from build123d import *

# Parameters (mm, degrees)
F0_R             = 45
F0_R_2           = 33
F1_DEPTH         = 17
F2_R             = 5
F3_DEPTH         = 0.5
F3_COPIES_COUNT  = 6
F6_DEPTH         = 10
F8_COUNT         = 6
F9_W             = 6
F9_H             = 9
F10_DEPTH        = 17
F10_COPIES_COUNT = 3
F12_DEPTH        = 10
F12_COPIES_COUNT = 3
F14_DEPTH        = 1
F14_COPIES_COUNT = 3


# Not quite as in the source:
# - a pattern or mirror of a feature is missing from the dataset's text; its kind, count and spacing are read off the source's solid
# - a feature names something its author has since deleted; it is built from what else it names


with BuildPart() as f1:
    # F0 (on Front) → F1 (new body)
    with BuildSketch(Plane.XZ):
        Circle(F0_R)
        Circle(F0_R_2, mode=Mode.SUBTRACT)
    extrude(amount=F1_DEPTH)

    # F2 (on Front) → F3 (cut)
    with BuildSketch(Plane.XZ):
        with Locations((0, 39)):
            Circle(F2_R)
    f3 = extrude(amount=F3_DEPTH, mode=Mode.SUBTRACT)

    # F3_copies: F3 ×6 about axis
    f3_copies_axis = Axis((0, 0, 0), (0, 1, 0))
    for i in range(1, F3_COPIES_COUNT):
        add(f3.rotate(f3_copies_axis, i * 360 / F3_COPIES_COUNT), mode=Mode.SUBTRACT)

    # F5 (on face) → F6 (cut)
    with BuildSketch(Plane.XZ.offset(17)):
        with BuildLine():
            Line((-30.5409561082, 12.5), (-43.2290411645, 12.5))
            ThreePointArc((-43.2290411645, 12.5), (-45, 0), (-43.2290411645, -12.5))
            Line((-43.2290411645, -12.5), (-30.5409561082, -12.5))
            ThreePointArc((-30.5409561082, -12.5), (-33, 0), (-30.5409561082, 12.5))
        make_face()
    f6 = extrude(amount=-F6_DEPTH, mode=Mode.SUBTRACT)

    # F8: F6 ×6 about axis
    f8_axis = Axis((0, -20.116, 0), (0, -1, 0))
    for i in range(1, F8_COUNT):
        add(f6.rotate(f8_axis, i * 360 / F8_COUNT), mode=Mode.SUBTRACT)

    # F9 (on face) → F10 (join)
    with BuildSketch(Plane.XZ.offset(7)):
        with Locations((42, 0)):
            Rectangle(F9_W, F9_H)
    f10 = extrude(amount=F10_DEPTH)

    # F10_copies: F10 ×3 about axis
    f10_copies_axis = Axis((0, 0, 0), (0, 1, 0))
    for i in range(1, F10_COPIES_COUNT):
        add(f10.rotate(f10_copies_axis, i * 360 / F10_COPIES_COUNT))

    # F11 (on face) → F12 (cut)
    with BuildSketch(Plane(origin=(0, 0, -4.5), x_dir=(1, 0, 0), z_dir=(0, 0, -1))):
        Polygon((39, 24), (39, 23.6), (43, 22), (43, 21), (41, 20), (41, 7), (44.7744346698, 7), (45, 7), (45, 24), align=None)
    f12 = extrude(amount=-F12_DEPTH, mode=Mode.SUBTRACT)

    # F12_copies: F12 ×3 about axis
    f12_copies_axis = Axis((0, 0, 0), (0, 1, 0))
    for i in range(1, F12_COPIES_COUNT):
        add(f12.rotate(f12_copies_axis, i * 360 / F12_COPIES_COUNT), mode=Mode.SUBTRACT)

    # F13 (on Top) → F14 (join, symmetric)
    with BuildSketch(Plane.XY):
        Polygon((37, -7), (39, -17), (39, -7), align=None)
    f14 = extrude(amount=F14_DEPTH, both=True)

    # F14_copies: F14 ×3 about axis
    f14_copies_axis = Axis((0, 0, 0), (0, 1, 0))
    for i in range(1, F14_COPIES_COUNT):
        add(f14.rotate(f14_copies_axis, i * 360 / F14_COPIES_COUNT))


solid = f1.part
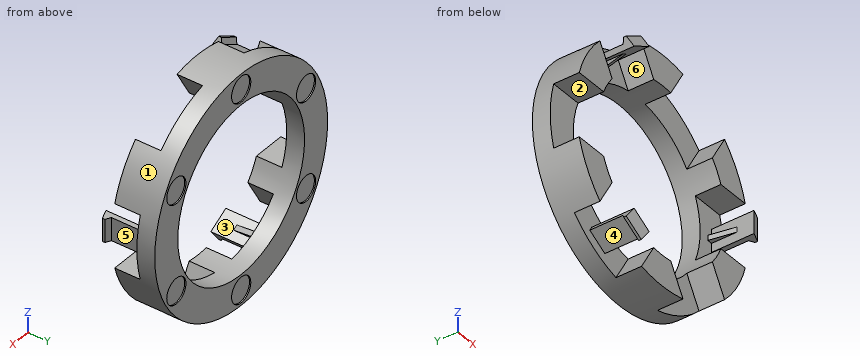
Source: CAD feature listing. Evaluate the final solid. Frame: model axes, mm. Face numbers are marked on the shaded views. A direction names the side the tool comes from. Give positions to 0.01 mm unless a question says otherwise; leave off trailing zeros. Order: outer loops, then holes, each group sorted by start corner. A loop starts at its lowest first (then second) coordinate and runs counter-clockwise, first axis right, second up. Notation, with made-up numbers: (57, -17.75) -> (105, -17.75) arc R23 ccw to (105, -6.75) -> close; hole circle Ø9 at (79.5, -8.75). An arc over 180 degrees is marked (long way). Write item = value, one per line.
Item 1: Ray query, probe 1 along Z at (x, y) = (0, -0.05); probe 2 along Y at (x, z) = (29, -30.5); probe 3 along Z at (x, y) = (17, -2.5). Return the intervals inside material, ascending.
Check result:
probe_1 = -45 to -44, -34 to -33, 33 to 34, 44 to 45
probe_2 = -7 to 0
probe_3 = -41.67 to -28.28, 28.28 to 41.67
Item 2: Section query B-B (z = -6.5). Output: boundary loops of the cut face in (x, y), then the cut area to 3 significant figures.
Check result:
outline = (-44.53, -7) -> (-32.35, -7) -> (-32.35, 0) -> (-44.53, 0) -> close; (32.35, -7) -> (44.53, -7) -> (44.53, 0) -> (32.35, 0) -> close
area = 170 mm²
Item 3: Set-up query: the marked faces 4, 5 and 6. Return all of +Z, -Z, +X, -X, +Y, -Y with unobstructed straight access to the full face (end or side cutting, diameter ignored); none if empty.
Check result:
face_4 = -Z, -X
face_5 = +X
face_6 = -Y
Item 4: Contact query for flat-ended pins moving along their axis: pin 1 (10 mm diameter, centred on x = -2, z = 40.5, fed in from -Y); pin 2 (3 mm diameter, centred on x = 41, y = -15.5, fed in from +Z); pin 3 (1 mm diameter, centred on x = -8.5, y = -16, fed in from +Z); pin 4 (11 mm diameter, centred on x = 1.5, z = -38.5, fed in from +Y). Output: stop coordinate, or through.
Check result:
pin_1 = -17
pin_2 = 21.56
pin_3 = 44.28
pin_4 = 0
Item 5: Mould query, pull axis X, two halves, no side actions, for the marked faces 1, 2 and 3. Classes: +X half, -X half, draft (parallel to the pull), parting line (faces both ways), or undercut.
Check result:
face_1 = parting line
face_2 = draft
face_3 = undercut
Item 6: Section query D-D (x = 23). Output: boundary loops of the cut face in (y, z).
Check result:
outline = (-7, -38.68) -> (0, -38.68) -> (0, -23.66) -> (-7, -23.66) -> close; (-7, 23.66) -> (0, 23.66) -> (0, 38.68) -> (-7, 38.68) -> close
Item 7: Section query A-A (x = 0). Output: boundary loops of the cut face in (y, z).
Check result:
outline = (-17, -45) -> (0, -45) -> (0, -44) -> (-0.5, -44) -> (-0.5, -34) -> (0, -34) -> (0, -33) -> (-17, -33) -> close; (-17, 33) -> (0, 33) -> (0, 34) -> (-0.5, 34) -> (-0.5, 44) -> (0, 44) -> (0, 45) -> (-17, 45) -> close
Item 8: Section query C-C (y = -5). Output: boundary loops of the cut face in (x, z).
Check result:
outline = circle Ø90 at (0, 0); hole circle Ø66 at (0, 0)
